Build history of the part. All positions in model axes, mm. A direction names the side the tool comes from. Coordinates: 2 decimals unless noted, no trailing zeros. Order: outer loops, then holes, each group sorted by start corner. A loop starts at its lowest first (then second) coordinate and runs counter-clockwise, first axis right, second up. Notation, with made-up numbers: (-27.75, 75) - (-11.75, 75) arc R19 ccw to (-11.75, 87) - close; hole circle Ø9 at (15, 34). An arc over 180 degrees is marked (long way). Write each question's results on one line, items separated by ' | '.
from build123d import *

# Parameters (mm, degrees)
SKETCH_W        = 32
SKETCH_H        = 40
PAD_DEPTH       = 7
SKETCH001_W     = 32
SKETCH001_H     = 40
SKETCH001_W_2   = 28
SKETCH001_H_2   = 36
PAD001_DEPTH    = 26
POCKET_DEPTH    = 5
SKETCH003_W     = 9
SKETCH003_H     = 4
POCKET001_DEPTH = 5


with BuildPart() as part:
    # Sketch → Pad (new body)
    with BuildSketch(Plane.XY):
        with Locations((16, 20)):
            Rectangle(SKETCH_W, SKETCH_H)
    extrude(amount=PAD_DEPTH)

    # Sketch001 → Pad001 (new body)
    with BuildSketch(Plane.XY.offset(7)):
        with Locations((16, 20)):
            Rectangle(SKETCH001_W, SKETCH001_H)
        with Locations((16, 20)):
            Rectangle(SKETCH001_W_2, SKETCH001_H_2, mode=Mode.SUBTRACT)
    extrude(amount=PAD001_DEPTH)

    # Sketch002 → Pocket (cut)
    with BuildSketch(Plane.XY.offset(7)):
        Polygon((3.5, 37.5), (28.5, 37.5), (28.5, 2.5), (16, 2.5), (3.5, 2.5), align=None)
    extrude(amount=-POCKET_DEPTH, mode=Mode.SUBTRACT)

    # Sketch003 → Pocket001 (cut)
    with BuildSketch(Plane.XZ):
        with Locations((16, 5)):
            Rectangle(SKETCH003_W, SKETCH003_H)
    extrude(amount=-POCKET001_DEPTH, mode=Mode.SUBTRACT)


solid = part.part
1. Drop flat-ended pins along their axis: pin 1 Ø14 at (x, y) = (9.5, 17) entering from +Z; pin 2 Ø12.5 at (x, y) = (15, 18) entering from +Z. Give the stop position or say it passes through.
Solved:
pin 1: stops at z = 7 | pin 2: stops at z = 2
2. Band-saw the part on A-A on x = 16. Give the cut face in (y, z), then the cut area to 3 significant figures.
Solved:
outline: (0, 0) - (40, 0) - (40, 33) - (38, 33) - (38, 7) - (37.5, 7) - (37.5, 2) - (2.5, 2) - (2.5, 3) - (0, 3) - close; (0, 7) - (2, 7) - (2, 33) - (0, 33) - close | area: 199 mm2
3. Tool access for faces 1 (the face through (20.5, 1, 5)), 2 (the face through (15.8, 2.5, 2.3)), 3 (the face through (1.7, 21.6, 33)): list every direction of +Z, -Z, +X, -X, +Y, -Y with a clear straight run to the whole face (end or side of a thin tool).
Solved:
face 1: -Y | face 2: +Z | face 3: +Z, +X, -X, +Y, -Y
4. Band-saw the part on C-C on y = 18.5. Give the cut face in (x, z).
Solved:
outline: (0, 0) - (32, 0) - (32, 33) - (30, 33) - (30, 7) - (28.5, 7) - (28.5, 2) - (3.5, 2) - (3.5, 7) - (2, 7) - (2, 33) - (0, 33) - close
5. Band-saw the part on D-D on z = 4. Give the cut face in (x, y), then the cut area to 4 significant figures.
Solved:
outline: (0, 0) - (11.5, 0) - (11.5, 2.5) - (3.5, 2.5) - (3.5, 37.5) - (28.5, 37.5) - (28.5, 2.5) - (20.5, 2.5) - (20.5, 0) - (32, 0) - (32, 40) - (0, 40) - close | area: 382.5 mm2
6. Two-plate mould, pull along X, no slides. Class faces 4 (the face through (16, 38, 20)), 5 (the face through (16, 40, 16)), 6 (the face through (3.5, 20, 5)), 7 (the face through (0, 20, 16)): +X half, -X half, draft (parallel to the pull), parting line (faces both ways), or undercut.
Solved:
face 4: undercut | face 5: draft | face 6: undercut | face 7: -X half
7. Band-saw the part on B-B on z = 17.5. Give the cut face in (x, y).
Solved:
outline: (0, 0) - (32, 0) - (32, 40) - (0, 40) - close; hole (2, 2) - (30, 2) - (30, 38) - (2, 38) - close
8. Probe line 1 (X direction, y = 4.5, z = 19.5); line 2 (X direction, y = 33.5, z = 2.5); line 3 (Y direction, x = 4.5, z = 31.5). List the from-to ranges inside material, lowest first.
Solved:
line 1: x = 0 to 2, 30 to 32 | line 2: x = 0 to 3.5, 28.5 to 32 | line 3: y = 0 to 2, 38 to 40
